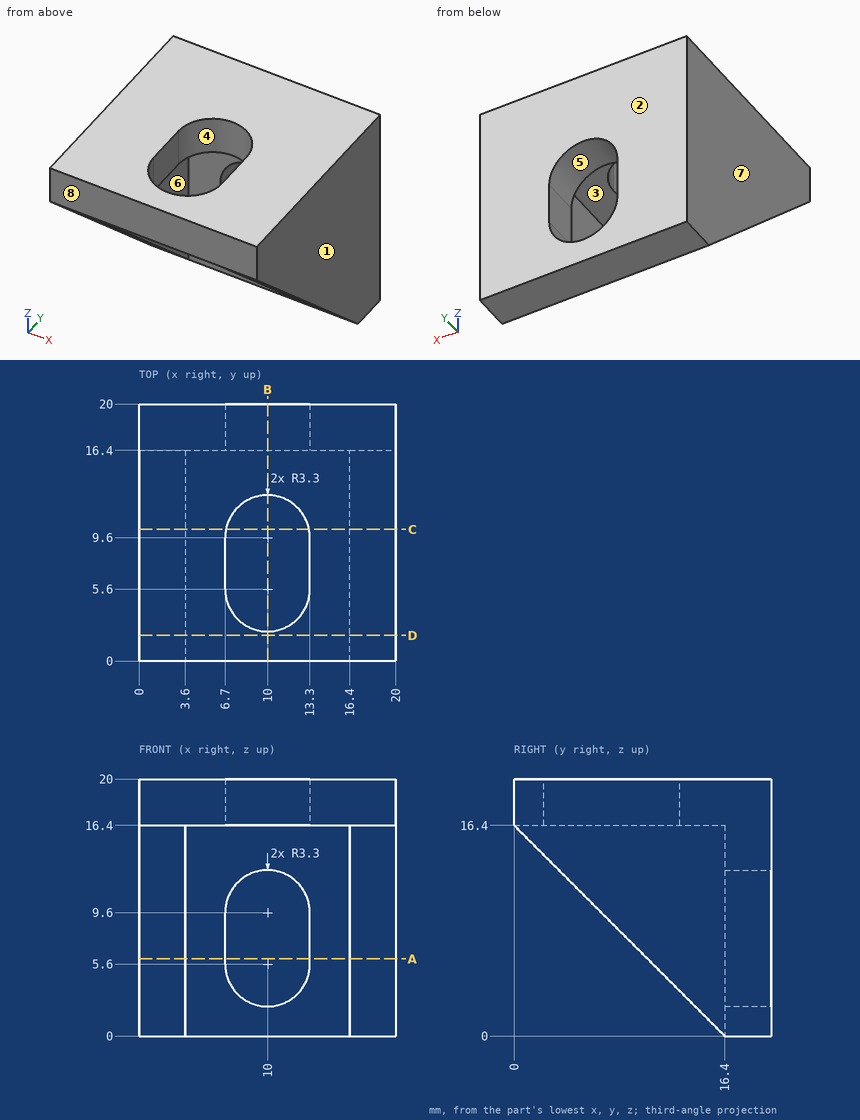
The figure shows three views and two pictorial views of one solid part (mm, origin at its lowest corner). Answer the questions. A direction names the side the tool comes from. Give positions to 0.01 mm unless a question says otherwise; leave off trailing zeros. Loops run counter-clockwise (first coordinate to the right, second up) from the corner with the lowest first, then second, coordinate; pieces in that order, holes last. Notation, with made-up numbers: (87, 28) -> (99, 28) arc R34 ccw to (99, 65) -> close; hole circle Ø2 at (37.25, 45.5). An arc over 180 degrees is marked (long way). Put each result on its own line as item: value. Start each with the question number.
Item 1: The mould has two halves that part along X. Classify the marked faces 6, 7 and 8: released by +X, released by -X, zero draft, split by the parting line, or undercut.
Item 2: Each of these flat-tipped pins is pushed along its axis until it touches: P1, Ø1, axis at x = 18, z = 8.5, coming from the -Y side; P2, Ø12, axis at x = 4.5, z = 9, coming from the -Y side. Where does it stop, or does it pass through?
Item 3: Which of the six approach directions +Z, -Z, +X, -X, +Y, -Y give full straight-line access (tool end or side, diameter ignored) to the marked faces 1, 2, 3, 4 and 5?
Item 4: The part is cut by section A-A (z = 6). Give the vertices of the cut face in (x, y), then the cut area to 3 significant figures.
Item 5: The part is cut by section C-C (y = 10.25). Give the vertices of the cut face in (x, z), then the cut area to 3 significant figures.
Item 6: Find the intervals of material crossed by L1, parallel to X at y = 19, z = 8.75; L2, parallel to X at y = 16, z = 4.5; L3, parallel to Y at x = 14.5, z = 12.5, in increasing order. Write a range as [from, to].
Item 7: The part is cut by section B-B (x = 10). Give the vertices of the cut face in (y, z).
Item 8: The part is cut by section D-D (y = 2). Give the vertices of the cut face in (x, z), then the cut area to 3 significant figures.
Answers below:
1. face 6: undercut
1. face 7: released by -X
1. face 8: zero draft
2. P1: y = 7.4
2. P2: y = 1.47
3. face 1: +Z, -Z, +X, +Y, -Y
3. face 2: +Z, -Z, +X, -X, +Y
3. face 3: -Z, -Y
3. face 4: +Z, -Z
3. face 5: +Y, -Y
4. outline: (0, 10.4) -> (3.6, 10.4) -> (3.6, 16.4) -> (6.7, 16.4) -> (6.7, 20) -> (0, 20) -> close; (13.3, 16.4) -> (16.4, 16.4) -> (16.4, 10.4) -> (20, 10.4) -> (20, 20) -> (13.3, 20) -> close
4. area: 91.4 mm2
5. outline: (0, 6.15) -> (3.6, 6.15) -> (3.6, 16.4) -> (6.76, 16.4) -> (6.76, 20) -> (0, 20) -> close; (13.24, 16.4) -> (16.4, 16.4) -> (16.4, 6.15) -> (20, 6.15) -> (20, 20) -> (13.24, 20) -> close
5. area: 123 mm2
6. L1: [0, 6.7], [13.3, 20]
6. L2: [0, 3.6], [16.4, 20]
6. L3: [16.4, 20]
7. outline: (0, 16.4) -> (2.3, 16.4) -> (2.3, 20) -> (0, 20) -> close; (12.9, 16.4) -> (16.4, 16.4) -> (16.4, 12.9) -> (20, 12.9) -> (20, 20) -> (12.9, 20) -> close; (16.4, 0) -> (20, 0) -> (20, 2.3) -> (16.4, 2.3) -> close
8. outline: (0, 14.4) -> (3.6, 14.4) -> (3.6, 16.4) -> (16.4, 16.4) -> (16.4, 14.4) -> (20, 14.4) -> (20, 20) -> (0, 20) -> close
8. area: 86.4 mm2
